Verification items for the finished model (mm, model axes). Round coordinates to 2 decimals unless told otherwise and drop trailing zeros. Write each loop counter-clockwise with the first axis right and the second up, starting at its lowest first coordinate (ties: lowest second). Pieces come first, ordered by that corner, then holes. Notation, with made-up numbers: M 5,38 L 29,38 A9 ccw 29,55 Z; hole C 76.5,66.25 d5. An arc over 180 degrees is marked long. One line per question, with ' | ' between items.
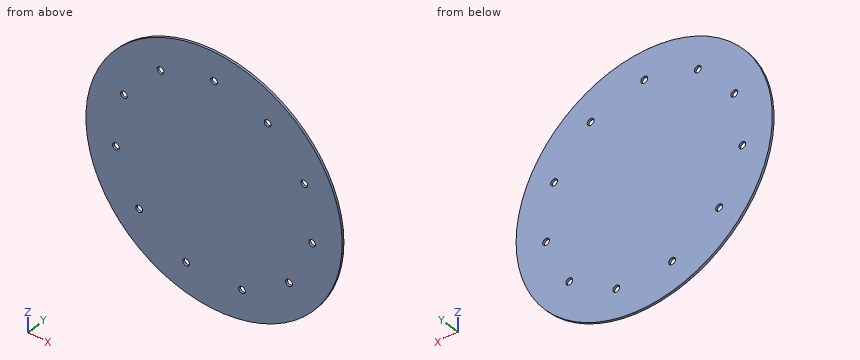
from build123d import *

# Parameters (mm, degrees)
F0_R            = 29.845
F1_DEPTH        = 0.508
F2_D            = 1.5875
F2_COPIES_COUNT = 11


# Not quite as in the source:
# - a pattern or mirror of a feature is missing from the dataset's text; its kind, count and spacing are read off the source's solid


with BuildPart() as f1:
    # F0 (on Front) → F1 (new body)
    with BuildSketch(Plane.XZ):
        Circle(F0_R)
    extrude(amount=F1_DEPTH)

    # F2 (through all)
    with Locations(Plane(origin=(0, 0, 0), x_dir=(1, 0, 0), z_dir=(0, 1, 0))):
        with Locations((0, -23.0886)):
            f2 = Hole(F2_D / 2)

    # F2_copies: F2 ×11 about axis
    f2_copies_axis = Axis((0, 0, 0), (0, 1, 0))
    for i in range(1, F2_COPIES_COUNT):
        add(f2.rotate(f2_copies_axis, i * 360 / F2_COPIES_COUNT), mode=Mode.SUBTRACT)


solid = f1.part
1. Thickness scan on line 1 (X direction, y = -0.3, z = -4); line 2 (Z direction, x = -0.5, y = -0.05); line 3 (Z direction, x = 13, y = -0.4). Record the ranges inside material, lowest first.
Results:
line 1: x = -29.58 to -23.2, -22.51 to 22.51, 23.2 to 29.58 | line 2: z = -29.84 to 22.47, 23.71 to 29.84 | line 3: z = -26.86 to 18.82, 20.03 to 26.86
2. Section check B-B, the plane y = -0.25. Count the separate pieces of the cut face and the enclosed holes in it, then the cut area to 3 significant figures.
Results:
separate pieces: 1 | enclosed holes: 11 | area: 2,780 mm2
3. Section check C-C, the plane x = 6.5. Record the cut outline in (y, z).
Results:
outline: M -0.51,-29.13 L 0,-29.13 L 0,-22.95 L -0.51,-22.95 Z; M -0.51,-21.36 L 0,-21.36 L 0,29.13 L -0.51,29.13 Z
4. Section check D-D, the plane z = -19.5. Record the cut outline in (x, y), then the cut area to 3 significant figures.
Results:
outline: M -22.59,-0.51 L 22.59,-0.51 L 22.59,0 L -22.59,0 Z | area: 23.0 mm2
5. Go/stop test with a flat-tipped pin: P1, Ø1.3, axis at x = 12.48, z = 19.42, coming from the +Y side. Record where the tip stops, or that it passes through.
Results:
P1: passes through
6. Section check A-A, the plane x = 0. Record the cut outline in (y, z) (3 decimals), then the cut area to 3 significant figures.
Results:
outline: M -0.508,-29.845 L 0,-29.845 L 0,22.295 L -0.508,22.295 Z; M -0.508,23.882 L 0,23.882 L 0,29.845 L -0.508,29.845 Z | area: 29.5 mm2
